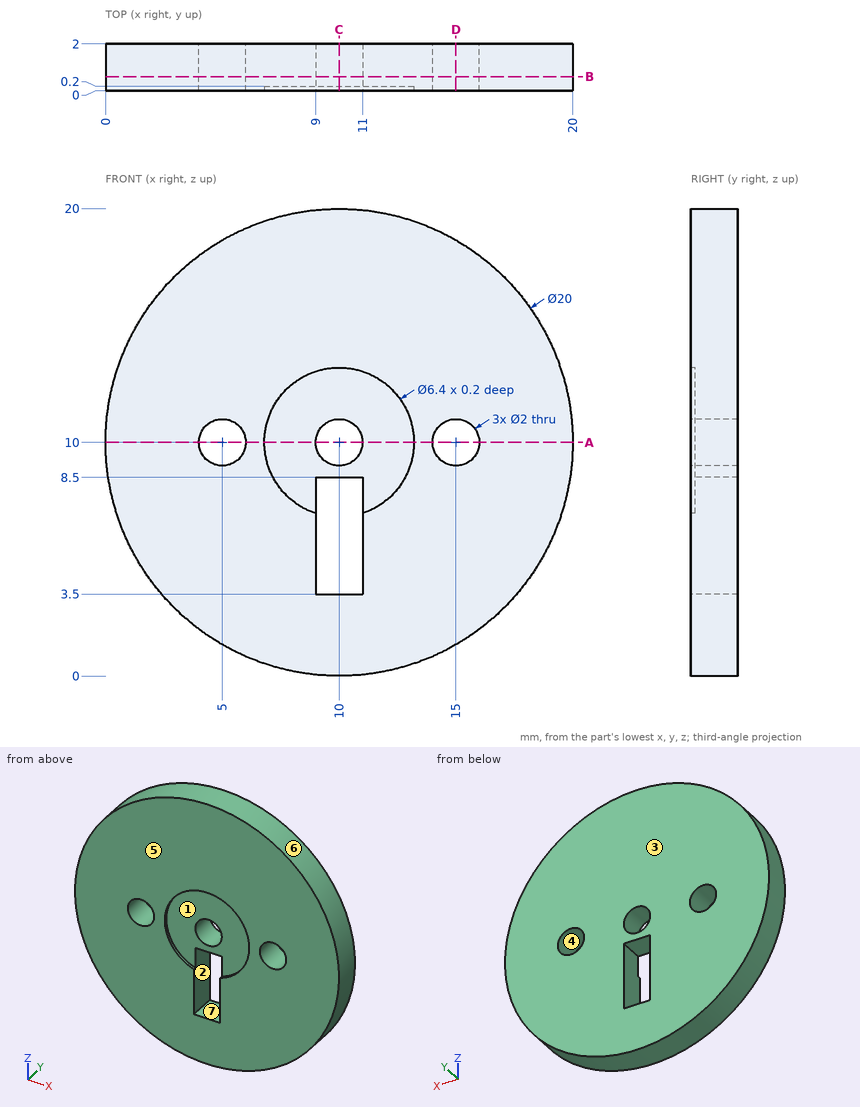
For this review, use the dimensioned drawing (mm, ordinates from the lowest corner) and the shaded views. A direction names the side the tool comes from. Round coordinates to 2 decimals unless told otherwise and drop trailing zeros. Write each loop counter-clockwise with the first axis right and the second up, starting at its lowest first coordinate (ties: lowest second). Pieces come first, ordered by that corner, then holes. Notation, with made-up numbers: (68, 19.25) -> (123, 19.25) arc R9 cw to (123, 36.25) -> close; hole circle Ø6 at (7.25, 55.5). An arc over 180 degrees is marked (long way). One line per item, written item: value. Start each with the question number.
Q1. To check wall thickness, follow probe 1 along X at (y, z) = (0.1, 10); probe 2 along X at (y, z) = (0.6, 10); probe 3 along Z at (x, y) = (4.25, 0.75). State the ranges of each line that lie inside material, in increasing order.
Q2. Insertion check: P1, Ø1, axis at x = 9, y = 1.5, coming from the +Z side; P2, Ø8, axis at x = 3, z = 17.5, coming from the -Y side; P3, Ø1, axis at y = 0.5, z = 14, coming from the -X side; P4, Ø1, axis at y = 1, z = 5, coming from the -X side. Each pin has a flat end and moves straight along its axis. Give the tip position at first contact, or say it passes through.
Q3. Add section A-A (z = 10). Give the boundary of the cut face in (x, y), then the cut area to 3 significant figures.
Q4. Add section D-D (x = 15). Give the boundary of the cut face in (y, z).
Q5. The part is to be moulded in two halves that separate along X. For the marked faces 4, 5, 6 and 7, say which applies: pulls with the +X half, pulls with the -X half, needs draft (parallel to the pull), parting line crosses it, or undercut.
Q6. Tool access review of the marked faces 1, 2 and 3: name each direction out of +Z, -Z, +X, -X, +Y, -Y from which nothing blocks a thin tool from reaching the whole face with its end or side.
Q7. Add section C-C (x = 10). Give the boundary of the cut face in (y, z).
Q8. Add section B-B (y = 0.6). Give the boundary of the cut face in (x, z).
Response:
1. probe 1: x = 0 to 4, 6 to 6.8, 13.2 to 14, 16 to 20
1. probe 2: x = 0 to 4, 6 to 9, 11 to 14, 16 to 20
1. probe 3: z = 1.82 to 9.34, 10.66 to 18.18
2. P1: stops at z = 19.99
2. P2: stops at y = 0
2. P3: stops at x = 0.63
2. P4: stops at x = 1.07
3. outline: (0, 0) -> (4, 0) -> (4, 2) -> (0, 2) -> close; (6, 0) -> (6.8, 0) -> (6.8, 0.2) -> (9, 0.2) -> (9, 2) -> (6, 2) -> close; (11, 0.2) -> (13.2, 0.2) -> (13.2, 0) -> (14, 0) -> (14, 2) -> (11, 2) -> close; (16, 0) -> (20, 0) -> (20, 2) -> (16, 2) -> close
3. area: 27.1 mm^2
4. outline: (0, 1.34) -> (2, 1.34) -> (2, 9) -> (0, 9) -> close; (0, 11) -> (2, 11) -> (2, 18.66) -> (0, 18.66) -> close
5. face 4: undercut
5. face 5: needs draft
5. face 6: parting line crosses it
5. face 7: undercut
6. face 1: -Y
6. face 2: +Y, -Y
6. face 3: +Z, -Z, +X, -X, +Y
7. outline: (0, 0) -> (2, 0) -> (2, 3.5) -> (0, 3.5) -> close; (0, 13.2) -> (0.2, 13.2) -> (0.2, 11) -> (2, 11) -> (2, 20) -> (0, 20) -> close; (0.2, 8.5) -> (2, 8.5) -> (2, 9) -> (0.2, 9) -> close
8. outline: circle Ø20 at (10, 10); hole circle Ø2 at (5, 10); hole (9, 3.5) -> (11, 3.5) -> (11, 8.5) -> (9, 8.5) -> close; hole circle Ø2 at (10, 10); hole circle Ø2 at (15, 10)
